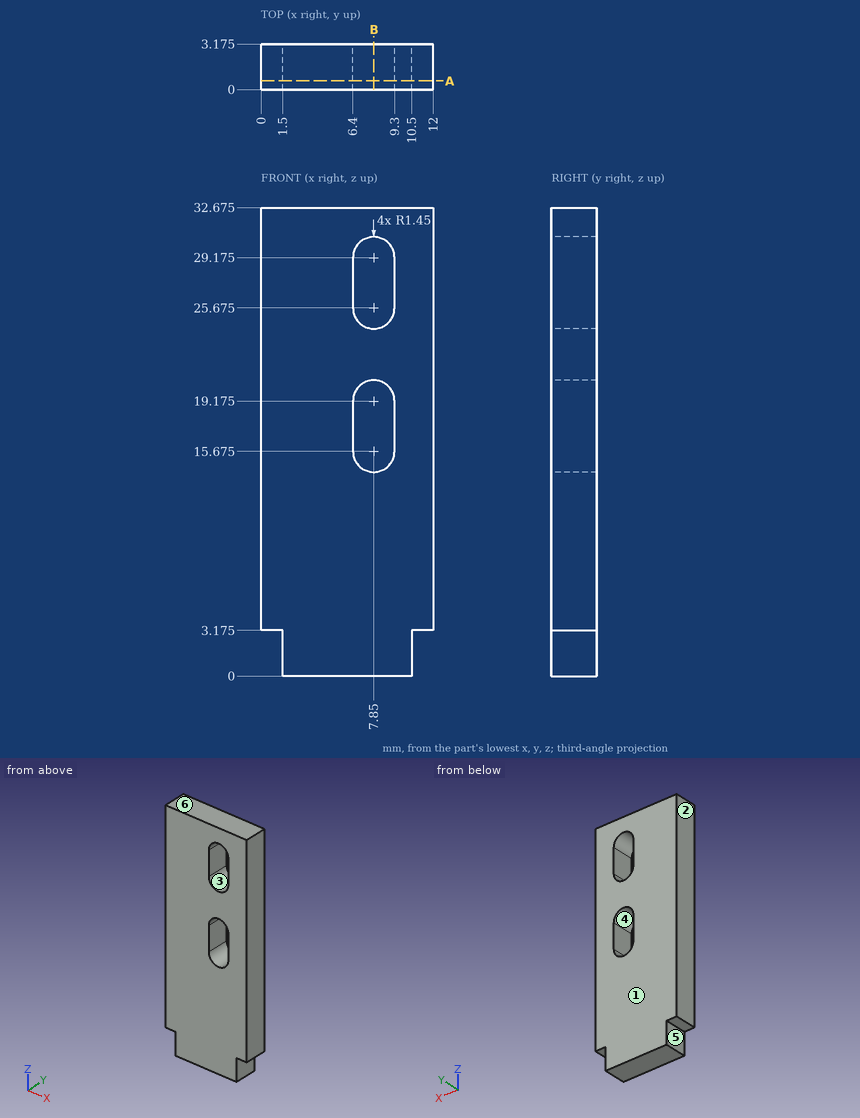
Design review of the part shown in the three views and the two pictorial views. Dimensions are in mm from the part's minimum x, y and z. A direction names the side the tool comes from. Give positions to 0.01 mm unless a question says otherwise; leave off trailing zeros. Loops run counter-clockwise (first coordinate to the right, second up) from the corner with the lowest first, then second, coordinate; pieces in that order, holes last. Notation, with made-up numbers: M 34.5,-36 L 85.5,-36 A21 ccw 85.5,-8 Z; hole C 40,85.25 d4. An arc over 180 degrees is marked long. Put each result on its own line as item: value. Start each with the question number.
(1) Wall thickness on L1, parallel to Z at x = 7.75, y = 1.5 (3 decimals); L2, parallel to X at y = 2.8, z = 29; L3, parallel to Z at x = 7.5, y = 1.05 (3 decimals): over which ranges is each line inside the solid? List them lowest first.
(2) Machinability: for the marked faces 4, 5 and 6, which of the approach directions +Z, -Z, +X, -X, +Y, -Y give a long, thin tool a straight path to every point of the face, cutting with its end or side? Answer none if there is none.
(3) Add section B-B, the plane x = 7.85. Write out the cut boundary in (y, z) (3 decimals), then the cut area to 3 significant figures.
(4) The part is to be moulded in two halves that separate along X. For the marked faces 1, 2 and 3, say which applies: +X half, -X half, draft (parallel to the pull), parting line (faces both ways), or undercut.
(5) Add section A-A, the plane y = 0.6. Write out the cut boundary in (x, z) (3 decimals).
(6) For pin 1 (0.8 mm diameter, centred on x = 1, y = 1, fed in from -Z) (3 decimals); pin 2 (1.6 mm diameter, centred on y = 2, z = 1, fed in from +X), all flat-tipped, find the tip position at first contact; note any pin that passes through.
Result:
1. L1: z = 0 to 14.228, 20.622 to 24.228, 30.622 to 32.675
1. L2: x = 0 to 6.4, 9.3 to 12
1. L3: z = 0 to 14.268, 20.582 to 24.268, 30.582 to 32.675
2. face 4: +Y, -Y
2. face 5: -Z, -X, +Y, -Y
2. face 6: +Z, +X, -X, +Y, -Y
3. outline: M 0,0 L 3.175,0 L 3.175,14.225 L 0,14.225 Z; M 0,20.625 L 3.175,20.625 L 3.175,24.225 L 0,24.225 Z; M 0,30.625 L 3.175,30.625 L 3.175,32.675 L 0,32.675 Z
3. area: 63.1 mm^2
4. face 1: draft
4. face 2: -X half
4. face 3: undercut
5. outline: M 0,3.175 L 1.5,3.175 L 1.5,0 L 10.5,0 L 10.5,3.175 L 12,3.175 L 12,32.675 L 0,32.675 Z; hole M 6.4,15.675 A1.45 ccw 9.3,15.675 L 9.3,19.175 A1.45 ccw 6.4,19.175 Z; hole M 6.4,25.675 A1.45 ccw 9.3,25.675 L 9.3,29.175 A1.45 ccw 6.4,29.175 Z
6. pin 1: stops at z = 3.175
6. pin 2: stops at x = 10.5
